Part model, mm, in its own coordinate system. Round coordinates to 2 decimals unless told otherwise and drop trailing zeros. Loops run counter-clockwise (first coordinate to the right, second up) from the corner with the lowest first, then second, coordinate; pieces in that order, holes last. Notation, with made-up numbers: (88.5, -16.5) - (132.5, -16.5) arc R21 cw to (132.5, 1.5) - close; hole circle Ø7 at (71, -31.75). An arc over 180 degrees is marked (long way). Write each question's results on one line, items separated by ' | '. Start each with the question number.
(1) Cut at A-A, the plane z = -3.81. List the corners of the cut face in (x, y).
(2) Drill centre lines: L1, parallel to Z at x = -5.5, y = 0.4; L2, parallel to X at y = 0.6, z = 8.5; L3, parallel to X at y = 0.45, z = 6.5. Where is each one in solid material? Low to high.
(3) Cut at B-B, the plane y = 1.2. Give the number of separate pieces and of enclosed holes in the cut face, then the cut area to 3 significant figures.
(4) Flat gauge pin, fed straight in: P1, Ø4, axis at x = -5.5, z = -10.25, coming from the +Y side. Where does the tip first touch, or does it go through?
Autodesk Inventor part; units mm, degrees
ref_plane "YZ Plane" through (0, 0, 0) normal (1, 0, 0) x (0, 1, 0)
ref_plane "XZ Plane" through (0, 0, 0) normal (0, 1, 0) x (-1, 0, 0)
ref_plane "XY Plane" through (0, 0, 0) normal (0, 0, 1) x (1, 0, 0)
sketch "Sketch1" plane through (0, 0, 0) normal (0, 1, 0) x (-1, 0, 0)
  line L0 (7.5, -12.5) -> (-7.5, -12.5)
  line L1 (-7.5, -12.5) -> (-7.5, 12.5)
  line L2 (-7.5, 12.5) -> (7.5, 12.5)
  line L3 (7.5, 12.5) -> (7.5, -12.5)
  line L4 (7.5, -12.5) -> (-7.5, 12.5) construction
  line L5 (-7.5, -12.5) -> (7.5, 12.5) construction
  circle A0 centre (5.5, 10.25) radius 1.5
  circle A1 centre (5.5, -10.25) radius 1.5
  line L6 (-6, 12.5) -> (-6, -12.5) construction
  circle A2 centre (-6, 11.43) radius 0.5
  circle A3 centre (-6, 8.89) radius 0.5
  circle A4 centre (-6, 6.35) radius 0.5
  circle A5 centre (-6, 3.81) radius 0.5
  circle A6 centre (-6, 1.27) radius 0.5
  circle A7 centre (-6, -1.27) radius 0.5
  circle A8 centre (-6, -3.81) radius 0.5
  circle A9 centre (-6, -6.35) radius 0.5
  circle A10 centre (-6, -8.89) radius 0.5
  circle A11 centre (-6, -11.43) radius 0.5
  point P0 (0, 0)
  dimension "d0" = 15
  dimension "d1" = 25
  dimension "d2" = 3
  dimension "d3" = 2.25
  dimension "d4" = 3
  dimension "d5" = 20.5
  dimension "d6" = 2.25
  dimension "d7" = 2
  dimension "d8" = 2
  dimension "d11" = 1.5
  dimension "d12" = 1
  dimension "d13" = 1.07
  dimension "d16" = 2.54
  dimension "d21" = 1.07
extrude "Extrusion2" add sketch "Sketch1" along normal blind 1.57
properties part number "board"
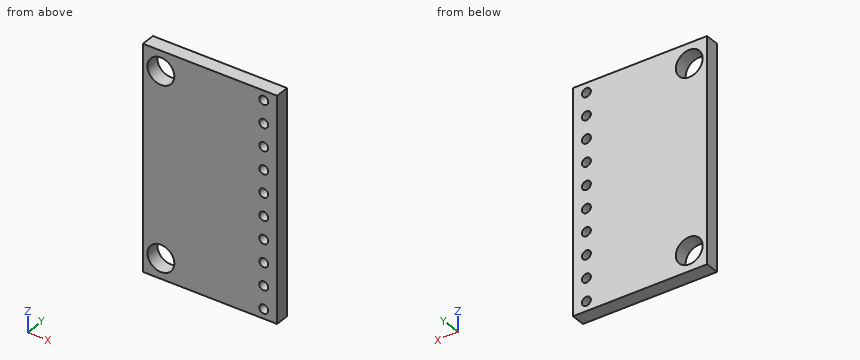
A:
1) outline: (-7.5, 0) - (5.5, 0) - (5.5, 1.57) - (-7.5, 1.57) - close; (6.5, 0) - (7.5, 0) - (7.5, 1.57) - (6.5, 1.57) - close
2) L1: -12.5 to -11.75, -8.75 to 8.75, 11.75 to 12.5 | L2: -7.5 to 5.69, 6.31 to 7.5 | L3: -7.5 to 5.52, 6.48 to 7.5
3) separate pieces: 1 | enclosed holes: 12 | area: 353 mm2
4) P1: y = 1.57
